```python
from build123d import *

# Parameters (mm, degrees)
SCHIZZO2_R                   = 20.9
ESTRUSIONE_ESTRUSIONE1_DEPTH = 10.75
SCHIZZO3_R                   = 3
ESTRUSIONE_ESTRUSIONE2_DEPTH = 8
SMUSSO1_SIZE                 = 5
SMUSSO1_SIZE2                = 8.660254038


with BuildPart() as part:
    # Schizzo2 → Estrusione-Estrusione1 (new body, symmetric)
    with BuildSketch(Plane.XY):
        Circle(SCHIZZO2_R)
    extrude(amount=ESTRUSIONE_ESTRUSIONE1_DEPTH, both=True)

    # Schizzo3 → Estrusione-Estrusione2 (add)
    with BuildSketch(Plane(origin=(0, 0, -10.75), x_dir=(-1, 0, 0), z_dir=(0, 0, -1))):
        Circle(SCHIZZO3_R)
    extrude(amount=ESTRUSIONE_ESTRUSIONE2_DEPTH)

    # Smusso1
    smusso1_edges = [part.edges().sort_by_distance(p)[0] for p in [
        (-20.9, 0, -10.75),
        (-20.9, 0, 10.75),
    ]]
    smusso1_side = [part.faces().sort_by_distance(p)[0] for p in [
        (-20.9, 0, 0),
    ]]
    chamfer(smusso1_edges, length=SMUSSO1_SIZE, length2=SMUSSO1_SIZE2, reference=smusso1_side[0])


solid = part.part
```
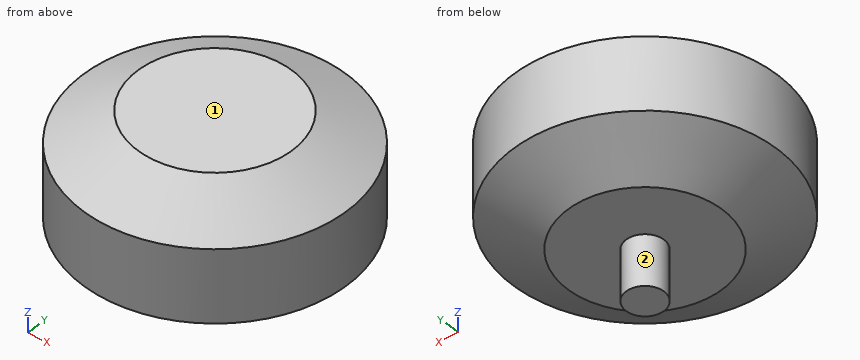
Model file for the job. Use its own axes, mm. Face numbers are marked on the shaded views. A direction names the side the tool comes from. Give positions to 0.01 mm unless a question says otherwise; leave off trailing zeros. Order: outer loops, then holes, each group sorted by start corner. A loop starts at its lowest first (then second) coordinate and runs counter-clockwise, first axis right, second up.
1) Saw through at A-A, the plane x = 0. Write the cut outline in (y, z).
2) Saw through at C-C, the plane z = -16. Write the cut outline in (x, y), then the cut area to 3 significant figures.
3) Pin check, flat tips, straight feed: pin 1 (8 mm diameter, centred on x = -7, z = 1.5, fed in from -Y); pin 2 (5 mm diameter, centred on x = -15, z = 4, fed in from +Y); pin 3 (5 mm diameter, centred on y = -11.5, z = -3, fed in from -X); pin 4 (4 mm diameter, centred on x = 7.5, z = -13.5, fed in from +Y). Stop position of each tip, or through.
4) Saw through at D-D, the plane z = -3. Write the cut outline in (x, y), then the cut area to 3 significant figures.
5) 3-axis set-ups, long thin cutter, end or side, ignore diameter. For the marked faces 1 and 2: which of +Z, -Z, +X, -X, +Y, -Y reach the whole face in a straight line?
6) Wall check: probe 1 along Z at (x, y) = (5.5, -5.5); probe 2 along X at (y, z) = (16.5, 4.25); probe 3 along X at (y, z) = (7, -4). Give the ranges that are in metal, low to high.
Computed:
1. outline: (-20.9, -5.75) - (-12.24, -10.75) - (-3, -10.75) - (-3, -18.75) - (3, -18.75) - (3, -10.75) - (12.24, -10.75) - (20.9, -5.75) - (20.9, 5.75) - (12.24, 10.75) - (-12.24, 10.75) - (-20.9, 5.75) - close
2. outline: circle Ø6 at (0, 0)
2. area: 28.3 mm2
3. pin 1: stops at y = -20.68
3. pin 2: stops at y = 16.75
3. pin 3: stops at x = -18.86
3. pin 4: passes through
4. outline: circle Ø41.8 at (0, 0)
4. area: 1,370 mm2
5. face 1: +Z, +X, -X, +Y, -Y
5. face 2: -Z
6. probe 1: z = -10.75 to 10.75
6. probe 2: x = -12.83 to 12.83
6. probe 3: x = -19.69 to 19.69
